from build123d import *

# Parameters (mm, degrees)
F1_DEPTH = 1.2
F2_DEPTH = 4
F3_R     = 0.85
F4_DEPTH = 1.5


with BuildPart() as f1:
    # F0 (on Front) → F1 (new body)
    with BuildSketch(Plane.XZ):
        Polygon((-2.354259, 13.55), (-7.034259, -15.25), (-5.210649, -15.25), (-0.823149, 11.75), (0.823149, 11.75), (5.210649, -15.25), (7.034259, -15.25), (2.354259, 13.55), align=None)
    extrude(amount=F1_DEPTH)

    # F0 (on Front) → F2 (join)
    with BuildSketch(Plane.XZ):
        Polygon((0, 14.75), (-3.375, 14.75), (-8.25, -15.25), (-7.034259, -15.25), (-2.354259, 13.55), (2.354259, 13.55), (7.034259, -15.25), (8.25, -15.25), (3.375, 14.75), align=None)
    extrude(amount=F2_DEPTH)

    # F3 (on face) → F4 (cut)
    with BuildSketch(Plane.XY.offset(14.75)):
        with Locations((0, -2.191013)):
            Circle(F3_R)
    extrude(amount=-F4_DEPTH, mode=Mode.SUBTRACT)


solid = f1.part
Source: CAD feature listing. Evaluate the final solid. Frame: model axes, mm. A direction names the side the tool comes from. Give positions to 0.01 mm unless a question says otherwise; leave off trailing zeros. Write each loop counter-clockwise with the first axis right and the second up, starting at its lowest first coordinate (ties: lowest second). Pieces come first, ordered by that corner, then holes. Notation, with made-up numbers: (59, 65) -> (70, 65) arc R17 ccw to (70, 73) -> close; hole circle Ø10 at (75, 42.25). An arc over 180 degrees is marked (long way). Write item = value, one per line.
Q1. First-contact query: pin 1 (2 mm diameter, centred on x = 4.5, z = -5, fed in from +Y); pin 2 (1 mm diameter, centred on y = -2, z = 3, fed in from +X); pin 3 (1.3 mm diameter, centred on x = 0, y = -0.5, fed in from -Z); pin 4 (1 mm diameter, centred on x = 0, y = -2.19, fed in from -Z). Flat tips, straight axial feed; report the tip coordinate or a pass-through.
Here are the results:
pin_1 = 0
pin_2 = 5.37
pin_3 = 11.75
pin_4 = through
Q2. Mould query, pull axis X, two halves, no side actions, for faces 4 (the face through (-4.727, -2.58, -1.052)), 5 (the face through (-5.78, -1.97, -0.04)), 6 (the face through (7.4, -1.5, -15.25)), 7 (the face through (3.1, -1.2, -0.8)). Classes: +X half, -X half, draft (parallel to the pull), parting line (faces both ways), or undercut.
Here are the results:
face_4 = undercut
face_5 = -X half
face_6 = draft
face_7 = undercut
Q3. Cut plane B-B on z = -6. Return loops of the section in (x, y).
Here are the results:
outline = (-6.75, -4) -> (-5.53, -4) -> (-5.53, -1.2) -> (-3.71, -1.2) -> (-3.71, 0) -> (-6.75, 0) -> close; (3.71, -1.2) -> (5.53, -1.2) -> (5.53, -4) -> (6.75, -4) -> (6.75, 0) -> (3.71, 0) -> close
Q4. Line query: line 1 (Y direction, x = 0, z = 14.5); line 2 (X direction, y = -0.95, z = 3.5); line 3 (X direction, y = -1.4, z = -9.5). Output: solid intervals per line, ascending. Write a range as from..to.
Here are the results:
line_1 = -4..-3.04, -1.34..0
line_2 = -5.2..-2.16, 2.16..5.2
line_3 = -7.32..-6.1, 6.1..7.32
Q5. Cut plane A-A on x = 0. Return loops of the section in (y, z), then the cut area to 3 significant figures.
Here are the results:
outline = (-4, 13.55) -> (-3.04, 13.55) -> (-3.04, 14.75) -> (-4, 14.75) -> close; (-1.34, 13.55) -> (-1.2, 13.55) -> (-1.2, 11.75) -> (0, 11.75) -> (0, 14.75) -> (-1.34, 14.75) -> close
area = 4.92 mm²
Q6. Cut plane D-D on y = -0.9. Return loops of the section in (x, z) (3 decimals), then the cut area to 3 significant figures.
Here are the results:
outline = (-8.25, -15.25) -> (-5.211, -15.25) -> (-0.823, 11.75) -> (0.823, 11.75) -> (5.211, -15.25) -> (8.25, -15.25) -> (3.375, 14.75) -> (-3.375, 14.75) -> close
area = 186 mm²
Q7. Cut plane C-C on y = -2.6. Return loops of the section in (x, z) (3 decimals), then the cut area to 3 significant figures.
Here are the results:
outline = (-8.25, -15.25) -> (-7.034, -15.25) -> (-2.354, 13.55) -> (-0.745, 13.55) -> (-0.745, 14.75) -> (-3.375, 14.75) -> close; (0.745, 13.55) -> (2.354, 13.55) -> (7.034, -15.25) -> (8.25, -15.25) -> (3.375, 14.75) -> (0.745, 14.75) -> close
area = 76.6 mm²
Q8. Reachability of faces 1 (the face through (2.986, -0.592, -1.561)), 2 (the face through (5.847, -1.972, -0.46)), 3 (the face through (4.66, -2.58, -0.65)) from +Z, -Z, +X, -X, +Y, -Y: full face, straight path, thin tool, end or side. Return the list, or none.
Here are the results:
face_1 = -Z, +Y, -Y
face_2 = +Z, +X, +Y, -Y
face_3 = -Z, -Y
